```python
from build123d import *

# Parameters (mm, degrees)
F0_W      = 180
F0_H      = 180
F1_DEPTH  = 70
F2_T      = -5
F3_W      = 170
F3_H      = 170
F4_DEPTH  = 10
F5_W      = 155
F5_H      = 155
F6_DEPTH  = 5
F7_W      = 145
F7_H      = 145
F8_DEPTH  = 25
F9_W      = 20
F9_H      = 20
F10_DEPTH = 5


with BuildPart() as f1:
    # F0 (on Top) → F1 (new body)
    with BuildSketch(Plane.XY):
        Rectangle(F0_W, F0_H)
    extrude(amount=F1_DEPTH)

    # F2
    f2_openings = [f1.faces().sort_by_distance(p)[0] for p in [
        (0, 0, 70),
    ]]
    offset(amount=F2_T, openings=f2_openings)

    # F3 (on face) → F4 (join)
    with BuildSketch(Plane.XY.offset(70)):
        Rectangle(F3_W, F3_H)
    extrude(amount=-F4_DEPTH)

    # F5 (on face) → F6 (cut)
    with BuildSketch(Plane.XY.offset(70)):
        Rectangle(F5_W, F5_H)
    extrude(amount=-F6_DEPTH, mode=Mode.SUBTRACT)

    # F7 (on face) → F8 (cut)
    with BuildSketch(Plane.XY.offset(65)):
        Rectangle(F7_W, F7_H)
    extrude(amount=-F8_DEPTH, mode=Mode.SUBTRACT)

    # F9 (on face) → F10 (join)
    with BuildSketch(Plane.XY.offset(65)):
        with Locations((-62.5, 62.5)):
            Rectangle(F9_W, F9_H)
        with Locations((62.5, 62.5)):
            Rectangle(F9_W, F9_H)
        with Locations((62.5, -62.5)):
            Rectangle(F9_W, F9_H)
        with Locations((-62.5, -62.5)):
            Rectangle(F9_W, F9_H)
    extrude(amount=-F10_DEPTH)


solid = f1.part
```
Work out the finished part from the listing and answer in its coordinate system (mm). A direction names the side the tool comes from. Give positions to 0.01 mm unless a question says otherwise; leave off trailing zeros. Loops run counter-clockwise (first coordinate to the right, second up) from the corner with the lowest first, then second, coordinate; pieces in that order, holes last. Notation, with made-up numbers: (48, 37.5) - (85, 37.5) arc R27 cw to (85, 64.5) - close; hole circle Ø3 at (34, 86.5). An arc over 180 degrees is marked (long way). One line per question, with ' | ' between items.
(1) Each of these flat-tipped pins is pushed along its axis until it touches: pin 1 Ø8 at (x, y) = (10, 16) entering from +Z; pin 2 Ø10 at (x, y) = (-49, 64.5) entering from +Z. Where does it stop, or does it pass through?
Recorded:
pin 1: stops at z = 5 | pin 2: stops at z = 65
(2) The part is cut by section A-A (z = 19). Write down the section's boundary in (x, y).
Recorded:
outline: (-90, -90) - (90, -90) - (90, 90) - (-90, 90) - close; hole (-85, -85) - (85, -85) - (85, 85) - (-85, 85) - close
(3) Straight lines are drawn through the part: probe 1 along X at (y, z) = (76.5, 23.5); probe 2 along Y at (x, z) = (64, 64). For each, find the intervals that lie inside material, in ascending order.
Recorded:
probe 1: x = -90 to -85, 85 to 90 | probe 2: y = -90 to -52.5, 52.5 to 90
(4) A tool of negligible diameter and unlimited length cuts with its end or side. For faces 3 (the face through (62, 52.5, 63)), 4 (the face through (-85, -1, 32)), from which of +Z, -Z, +X, -X, +Y, -Y can it reach the whole face along a straight path? Write none if from no direction.
Recorded:
face 3: +Z | face 4: none
(5) The mould has two halves that part along Y. Classify faces 1 (the face through (79, 1, 70)), 2 (the face through (52.5, -63, 63)): +Y half, -Y half, draft (parallel to the pull), parting line (faces both ways), or undercut.
Recorded:
face 1: draft | face 2: undercut
(6) The part is cut by section B-B (y = -63). Write down the section's boundary in (x, z), then the cut area to 3 significant figures.
Recorded:
outline: (-90, 0) - (90, 0) - (90, 70) - (77.5, 70) - (77.5, 65) - (52.5, 65) - (52.5, 60) - (85, 60) - (85, 5) - (-85, 5) - (-85, 60) - (-52.5, 60) - (-52.5, 65) - (-77.5, 65) - (-77.5, 70) - (-90, 70) - close | area: 1,950 mm²
